The listing builds one solid part. Answer for the finished solid, in the listing's coordinates (mm). A direction names the side the tool comes from. Coordinates: 2 decimals unless noted, no trailing zeros. Write each loop counter-clockwise with the first axis right and the second up, starting at its lowest first coordinate (ties: lowest second). Pieces come first, ordered by that corner, then holes. Notation, with made-up numbers: M -25.75,58 L -11.75,58 A24 ccw -11.75,90 Z; hole C 48.25,35.5 d1. An arc over 180 degrees is marked long. Answer as CSV lines item,"result".
```python
from build123d import *

# Parameters (mm, degrees)
F0_R     = 6.5
F1_DEPTH = 21
F2_R     = 0.5
F3_DEPTH = 10


with BuildPart() as f1:
    # F0 (on Top) → F1 (new body)
    with BuildSketch(Plane.XY):
        Circle(F0_R)
    extrude(amount=F1_DEPTH)

    # F2 (on Top) → F3 (join)
    with BuildSketch(Plane.XY):
        with Locations((-2.5, 0)):
            Circle(F2_R)
        with Locations((2.5, 0)):
            Circle(F2_R)
    extrude(amount=-F3_DEPTH)


solid = f1.part
```
Q1. For faces 1 (the flat face through (-2.5, 0, -10)), 2 (the cylindrical face through (-3, 0, -5)), determine the directions among +Z, -Z, +X, -X, +Y, -Y from which every point of the face is accessible in a straight line to the end or side of a thin tool.
Output:
face 1,"-Z, +X, -X, +Y, -Y"
face 2,"-Z"
Q2. Flat-ended cylindrical pins translate along their axes: pin 1 Ø1 at (y, z) = (1, 6.5) entering from -X; pin 2 Ø1.5 at (x, z) = (5, -0.5) entering from -Y; pin 3 Ø1 at (x, z) = (4, 10.5) entering from -Y. Find the tip coordinate at first contact, or state that the pin passes through.
Output:
pin 1,"x = -6.48"
pin 2,"y = -4.75"
pin 3,"y = -5.48"
Q3. Straight lines are drawn through the part: line 1 (Z direction, x = 0.25, y = -5); line 2 (Y direction, x = 2.5, z = -2); line 3 (Y direction, x = -2.5, z = 6.5). For each, find the intervals that lie inside material, in ascending order.
Output:
line 1,"0 to 21"
line 2,"-0.5 to 0.5"
line 3,"-6 to 6"
Q4. Find section D-D (z = 3.5). Give the vertices of the cut face in (x, y), and give its area (3 significant figures).
Output:
outline,"C 0,0 d13"
area,"133 mm2"
Q5. Find section C-C (z = -6). Give the vertices of the cut face in (x, y), and give its area (3 significant figures).
Output:
outline,"C -2.5,0 d1; C 2.5,0 d1"
area,"1.57 mm2"
Q6. Find section B-B (y = 0). Give the vertices of the cut face in (x, z).
Output:
outline,"M -6.5,0 L -3,0 L -3,-10 L -2,-10 L -2,0 L 2,0 L 2,-10 L 3,-10 L 3,0 L 6.5,0 L 6.5,21 L -6.5,21 Z"
Q7. Find section A-A (x = -2.5). Give the vertices of the cut face in (y, z), and give its area (3 significant figures).
Output:
outline,"M -6,0 L -0.5,0 L -0.5,-10 L 0.5,-10 L 0.5,0 L 6,0 L 6,21 L -6,21 Z"
area,"262 mm2"
